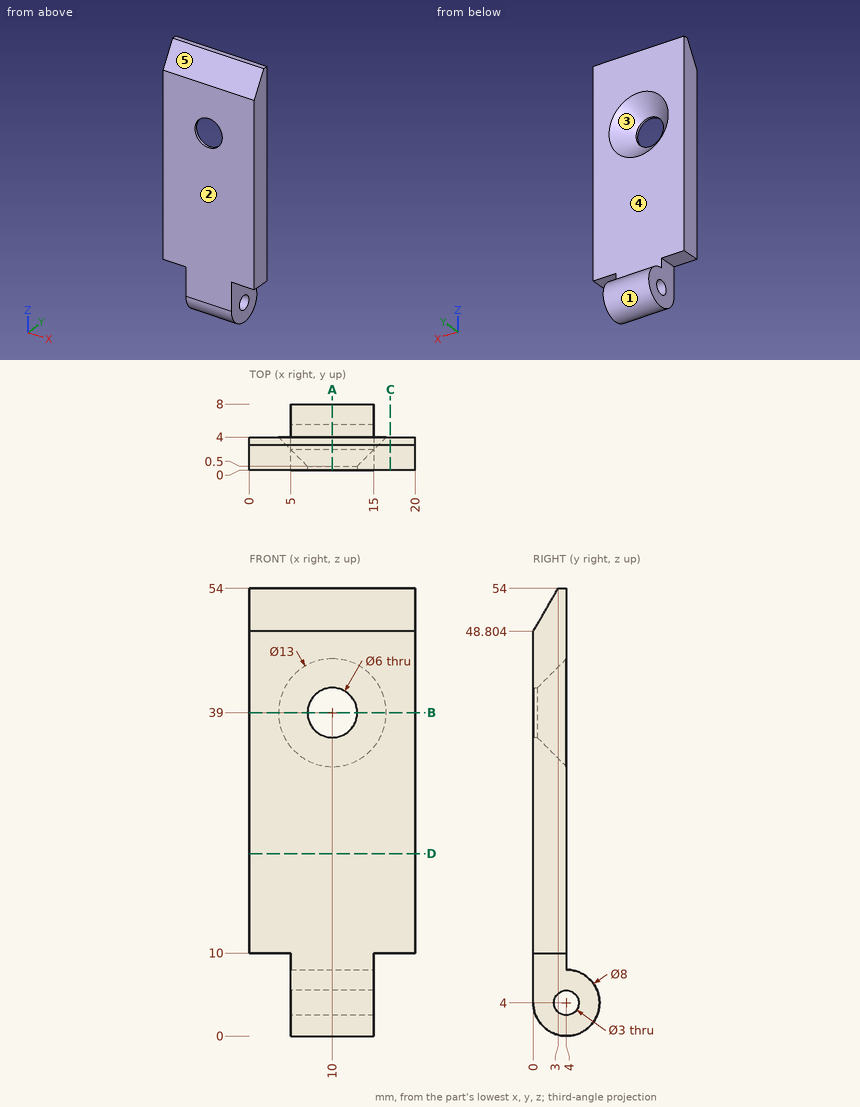
The drawing under review shows one solid part. Ordinate dimensions are in mm from its lowest x, y, z. A direction names the side the tool comes from. Give positions to 0.01 mm unless a question says otherwise; leave off trailing zeros. Loops run counter-clockwise (first coordinate to the right, second up) from the corner with the lowest first, then second, coordinate; pieces in that order, holes last. Notation, with made-up numbers: M 41,69 L 87,69 A19 cw 87,90 Z; hole C -17.5,80 d3. An arc over 180 degrees is marked long. One line per item, written item: value. Start each with the question number.
Q1. Add section C-C (x = 17). Give the boundary of the cut face in (y, z).
Q2. Add section B-B (z = 39). Give the boundary of the cut face in (x, y).
Q3. Draft analysis for pull direction Z (two halves, no side actions). For the marked faces 1, 2 and 3, state which applies: released by +Z, released by -Z, zero draft, split by the parting line, or undercut.
Q4. Add section D-D (z = 22). Give the boundary of the cut face in (x, y), and give its area (3 significant figures).
Q5. Add section A-A (x = 10). Give the boundary of the cut face in (y, z).
Q6. For L1, parallel to X at y = 0.25, z = 39; L2, parallel to Z at x = 13, y = 3.5 (1 decimal); L3, parallel to Y at x = 9.75, z = 45.5, list the stretches that pass through material, from the lowest coordinate up.
Q7. Machinability: for the marked faces 4 and 5, which of the approach directions +Z, -Z, +X, -X, +Y, -Y give a long, thin tool a straight path to every point of the face, cutting with its end or side? Answer none if there is none.
Q8. Clearance check with flat-ended pins moving along their axes: pin 1 Ø10 at (x, z) = (9, 36.5) entering from +Y; pin 2 Ø2 at (x, y) = (18, 2) entering from -Z; pin 3 Ø8 at (x, z) = (10, 39) entering from +Y. State where each tip first meets the part, or that it passes through.
Reply:
1. outline: M 0,10 L 4,10 L 4,54 L 3,54 L 0,48.8 Z
2. outline: M 0,0 L 7,0 L 7,0.5 L 3.5,4 L 0,4 Z; M 13,0 L 20,0 L 20,4 L 16.5,4 L 13,0.5 Z
3. face 1: split by the parting line
3. face 2: zero draft
3. face 3: undercut
4. outline: M 0,0 L 20,0 L 20,4 L 0,4 Z
4. area: 80.0 mm²
5. outline: M 0,4 A4 ccw long 4,8 L 4,32.5 L 0.5,36 L 0,36 Z; M 0,42 L 0.5,42 L 4,45.5 L 4,54 L 3,54 L 0,48.8 Z; hole C 4,4 d3
6. L1: 0 to 7, 13 to 20
6. L2: 0 to 2.6, 5.4 to 33.8, 44.2 to 54
6. L3: 0 to 4
7. face 4: +Z, +X, -X, +Y
7. face 5: +Z, +X, -X, -Y
8. pin 1: y = 4
8. pin 2: z = 10
8. pin 3: y = 1.5
